```python
from build123d import *

# Parameters (mm, degrees)
F0_W     = 67.058742
F0_H     = 27.341548
F1_DEPTH = 25.4
F2_W     = 14.965903
F2_H     = 14.678094
F3_DEPTH = 25.4
F4_R     = 7.396664
F5_DEPTH = 25.4
F6_W     = 14.390292
F6_H     = 15.253704
F7_DEPTH = 25.4


with BuildPart() as f1:
    # F0 (on Front) → F1 (new body)
    with BuildSketch(Plane.XZ):
        Rectangle(F0_W, F0_H)
    extrude(amount=F1_DEPTH)

    # F2 (on face) → F3 (cut)
    with BuildSketch(Plane.XZ.offset(25.4)):
        with Locations((-20.002499, 0)):
            Rectangle(F2_W, F2_H)
    extrude(amount=-F3_DEPTH, mode=Mode.SUBTRACT)

    # F4 (on face) → F5 (cut)
    with BuildSketch(Plane.XZ.offset(25.4)):
        Circle(F4_R)
    extrude(amount=-F5_DEPTH, mode=Mode.SUBTRACT)

    # F6 (on face) → F7 (cut)
    with BuildSketch(Plane.XZ.offset(25.4)):
        with Locations((20.002501, 0)):
            Rectangle(F6_W, F6_H)
    extrude(amount=-F7_DEPTH, mode=Mode.SUBTRACT)


solid = f1.part
```
Input: part model. Units: mm. Frame: model coordinates. A direction names the side the tool comes from. Coordinates: 2 decimals unless noted, no trailing zeros. Loops run counter-clockwise (first coordinate to the right, second up) from the corner with the lowest first, then second, coordinate; pieces in that order, holes last. Notation, with made-up numbers: (45, 80) - (55, 80) arc R22 cw to (55, 113) - close; hole circle Ø8 at (-28, 56.25). An arc over 180 degrees is marked (long way). Answer in a Markdown table with one row per item.
(1) Mould query, pull axis Z, two halves, no side actions, for faces 3 (the face through (-8, 0, 0)), 4 (the face through (20, -13, 7.627)), 5 (the face through (0, -13, -13.671)). Classes: pulls with the +Z half, pulls with the -Z half, needs draft (parallel to the pull), parting line crosses it, or undercut.
Model answer:
| item | result |
|---|---|
| face 3 | needs draft |
| face 4 | undercut |
| face 5 | pulls with the -Z half |
(2) Cut plane D-D on x = 23. Output: boundary loops of the cut face in (y, z), plus the area to 3 significant figures.
Model answer:
| item | result |
|---|---|
| outline | (-25.4, -13.67) - (0, -13.67) - (0, -7.63) - (-25.4, -7.63) - close; (-25.4, 7.63) - (0, 7.63) - (0, 13.67) - (-25.4, 13.67) - close |
| area | 307 mm² |
(3) Material intervals for L1, parallel to X at y = -11.5, z = -1.5; L2, parallel to X at y = -19, z = 3.75; L3, parallel to Z at x = -25, y = -17, sorted ascending. Write a range as from..to.
Model answer:
| item | result |
|---|---|
| L1 | x = -33.53..-27.49, -12.52..-7.24, 7.24..12.81, 27.2..33.53 |
| L2 | x = -33.53..-27.49, -12.52..-6.38, 6.38..12.81, 27.2..33.53 |
| L3 | z = -13.67..-7.34, 7.34..13.67 |
(4) Cut plane C-C on y = -8.5. Output: boundary loops of the cut face in (x, z).
Model answer:
| item | result |
|---|---|
| outline | (-33.53, -13.67) - (33.53, -13.67) - (33.53, 13.67) - (-33.53, 13.67) - close; hole (-27.49, -7.34) - (-12.52, -7.34) - (-12.52, 7.34) - (-27.49, 7.34) - close; hole circle Ø14.79 at (0, 0); hole (12.81, -7.63) - (27.2, -7.63) - (27.2, 7.63) - (12.81, 7.63) - close |
(5) Set-up query: faces 1 (the face through (-27.485, -13, 0)), 2 (the face through (33.529, -13, 0)). Return all of +Z, -Z, +X, -X, +Y, -Y with unobstructed straight access to the full face (end or side cutting, diameter ignored); none if empty.
Model answer:
| item | result |
|---|---|
| face 1 | +Y, -Y |
| face 2 | +Z, -Z, +X, +Y, -Y |
(6) Cut plane B-B on x = 0. Output: boundary loops of the cut face in (y, z).
Model answer:
| item | result |
|---|---|
| outline | (-25.4, -13.67) - (0, -13.67) - (0, -7.4) - (-25.4, -7.4) - close; (-25.4, 7.4) - (0, 7.4) - (0, 13.67) - (-25.4, 13.67) - close |
(7) Cut plane A-A on z = 0. Output: boundary loops of the cut face in (x, y), plus the area to 3 significant figures.
Model answer:
| item | result |
|---|---|
| outline | (-33.53, -25.4) - (-27.49, -25.4) - (-27.49, 0) - (-33.53, 0) - close; (-12.52, -25.4) - (-7.4, -25.4) - (-7.4, 0) - (-12.52, 0) - close; (7.4, -25.4) - (12.81, -25.4) - (12.81, 0) - (7.4, 0) - close; (27.2, -25.4) - (33.53, -25.4) - (33.53, 0) - (27.2, 0) - close |
| area | 582 mm² |
